Geometry check sheet. Reference: the model listing, model coordinates, mm. Round coordinates to 2 decimals unless told otherwise and drop trailing zeros. Write each loop counter-clockwise with the first axis right and the second up, starting at its lowest first coordinate (ties: lowest second). Pieces come first, ordered by that corner, then holes. Notation, with made-up numbers: M 89.5,83 L 105.5,83 A25 cw 105.5,98 Z; hole C 77.25,17 d2. An arc over 180 degrees is marked long. One line per item, written item: value. Start each with the question number.
1. Scan lines: probe 1 along Y at (x, z) = (98, 381); probe 2 along Y at (x, z) = (96, 381); probe 3 along Z at (x, y) = (94.75, -6.35). Record each from-to range of solid material in increasing order. Write a range as [from, to].
2. Depth check by flat-ended pin: P1, Ø5.5, axis at y = 379.65, z = 381, coming from the +X side; P2, Ø5.5, axis at y = -6.35, z = 381, coming from the -X side. Enter the tip coordinate at first touch or a pass-through.
3. Section check B-B (z = 154). Record the boundary of the cut face in (x, y).
4. Section check A-A (y = 341.5). Record the boundary of the cut face in (x, z).
5. Section check C-C (x = 55). Record the boundary of the cut face in (y, z).
from build123d import *

# Parameters (mm, degrees)
F1_DEPTH = 12.7
F2_W     = 12.7
F2_H     = 12.7
F3_DEPTH = 373.29999
F5_DEPTH = 12.7
F7_D     = 6.8
F7_DEPTH = 15.75
F7_TIP   = 2.0429261047
F9_D     = 5.1054
F9_DEPTH = 30.48
F9_TIP   = 1.5338169022


# Not quite as in the source:
# - a feature names something its author has since deleted; it is built from what else it names


with BuildPart() as f1:
    # F0 (on Front) → F1 (new body)
    with BuildSketch(Plane.XZ):
        Polygon((0, 25.4), (0, 0), (101.6, 0), (101.6, 387.3), (101.6, 400), (63.5, 400), align=None)
        Polygon((88.9, 387.3), (88.9, 12.7), (12.7, 12.7), (12.7, 25.4), (74.047170315, 387.3), align=None, mode=Mode.SUBTRACT)
    extrude(amount=F1_DEPTH)

    # F2 (on face) → F3 (join)
    with BuildSketch(Plane(origin=(0, 0, 0), x_dir=(-1, 0, 0), z_dir=(0, 1, 0))):
        with Locations((-95.25, 6.35)):
            Rectangle(F2_W, F2_H)
        with Locations((-95.25, 393.65)):
            Rectangle(F2_W, F2_H)
        Polygon((-12.7, 20.574), (-12.7, 12.7), (-12.7, 7.874), (0, 7.874), (0, 20.574), align=None)
        with Locations((-95.25, 380.95)):
            Rectangle(F2_W, F2_H)
    extrude(amount=F3_DEPTH)

    # F4 (on face) → F5 (join)
    with BuildSketch(Plane(origin=(0, 373.29999, 0), x_dir=(-1, 0, 0), z_dir=(0, 1, 0))):
        Polygon((-101.6, 374.6), (-101.6, 12.7), (-88.9, 12.7), (-88.9, 239.3), (-88.9, 374.6), align=None)
        Polygon((-101.6, 12.7), (-101.6, 0), (0, 0), (0, 25.4), (-63.5, 400), (-88.9, 400), (-88.9, 387.3), (-74.047170315, 387.3), (-12.7, 25.4), (-12.7, 12.7), (-88.9, 12.7), align=None)
        Polygon((-101.6, 400), (-101.6, 374.6), (-88.9, 374.6), (-88.9, 387.3), (-88.9, 400), align=None)
    extrude(amount=F5_DEPTH)

    # F7
    with Locations(Plane.YZ.offset(101.6)):
        with Locations((-6.35, 19), (-6.35, 381), (379.64999, 381), (379.64999, 19)):
            Hole(F7_D / 2, depth=F7_DEPTH)
            with Locations((0, 0, -(F7_DEPTH + F7_TIP / 2))):  # 118° drill point
                Cone(0, F7_D / 2, F7_TIP, mode=Mode.SUBTRACT)

    # F9
    with Locations(Plane.XY.offset(400)):
        with Locations((95.25, 353.4243106842), (95.25, 19.8756793158)):
            Hole(F9_D / 2, depth=F9_DEPTH)
            with Locations((0, 0, -(F9_DEPTH + F9_TIP / 2))):  # 118° drill point
                Cone(0, F9_D / 2, F9_TIP, mode=Mode.SUBTRACT)


solid = f1.part
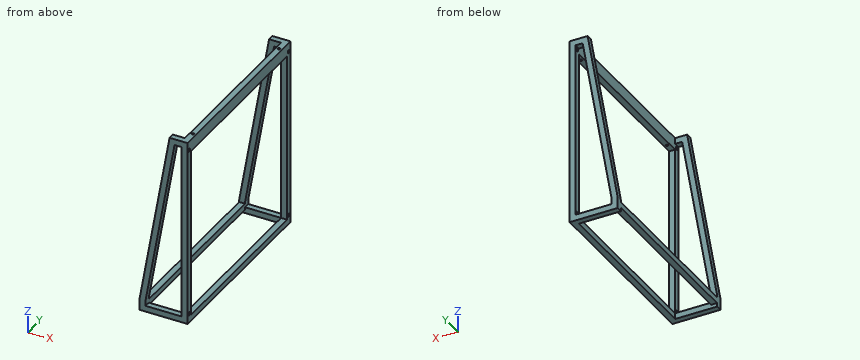
Result sheet:
1. probe 1: y = [-12.7, -9.75], [-2.95, 376.25], [383.05, 386]
1. probe 2: y = [-12.7, -9.75], [-2.95, 17.44], [22.32, 350.98], [355.86, 376.25], [383.05, 386]
1. probe 3: z = [0, 15.6], [22.4, 377.6], [384.4, 400]
2. P1: stops at x = 73.45
2. P2: stops at x = 59.81
3. outline: M 21.8,-12.7 L 34.5,-12.7 L 34.5,0 L 21.8,0 Z; M 21.8,373.3 L 34.5,373.3 L 34.5,386 L 21.8,386 Z; M 88.9,-12.7 L 101.6,-12.7 L 101.6,0 L 88.9,0 Z; M 88.9,373.3 L 101.6,373.3 L 101.6,386 L 88.9,386 Z
4. outline: M 0,7.87 L 12.7,7.87 L 12.7,20.57 L 0,20.57 Z; M 88.9,0 L 101.6,0 L 101.6,12.7 L 88.9,12.7 Z; M 88.9,374.6 L 101.6,374.6 L 101.6,400 L 88.9,400 Z
5. outline: M -12.7,0 L 0,0 L 0,12.7 L -12.7,12.7 Z; M -12.7,274.94 L 0,274.94 L 0,349.86 L -12.7,349.86 Z; M 373.3,0 L 386,0 L 386,12.7 L 373.3,12.7 Z; M 373.3,274.94 L 386,274.94 L 386,349.86 L 373.3,349.86 Z
